Source: three-view drawing plus pictorial views. Frame: mm from the lowest corner of the part. A direction names the side the tool comes from. Coordinates: 2 decimals unless noted, no trailing zeros. Order: outer loops, then holes, each group sorted by start corner. A loop starts at its lowest first (then second) coordinate and runs counter-clockwise, first axis right, second up. Notation, with made-up numbers: (-14.75, 34.25) -> (29.25, 34.25) arc R13 ccw to (29.25, 40.25) -> close; hole circle Ø1 at (78.5, 30). An arc over 180 degrees is marked (long way). One line per question, with ' | ' between items.
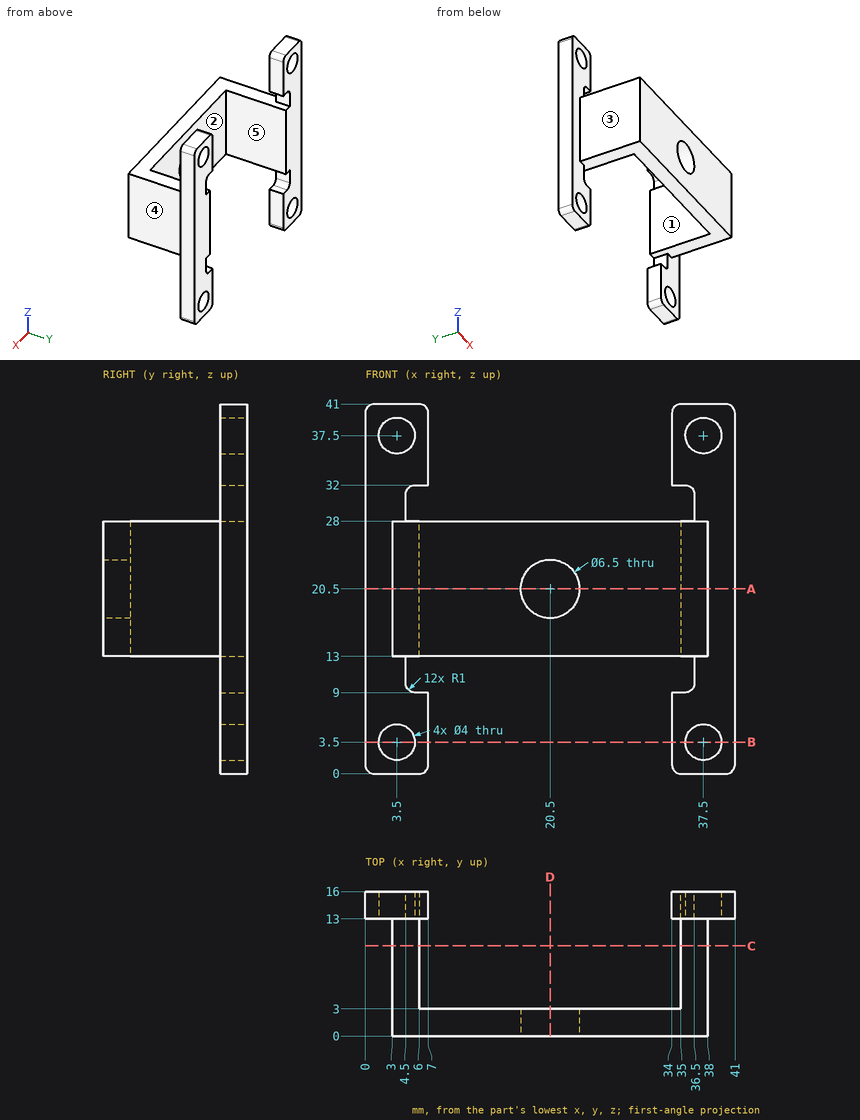
1. Cut plane C-C, the plane y = 10. Return loops of the section in (x, z).
Recorded:
outline: (3, 13) -> (6, 13) -> (6, 28) -> (3, 28) -> close; (35, 13) -> (38, 13) -> (38, 28) -> (35, 28) -> close
2. Access query for the marked faces 1, 2 and 3. Directions: +Z, -Z, +X, -X, +Y, -Y. A direction counts if a zero-diameter tool reaches every point of the face in a straight line with its end or side. Return the directions, or none.
Recorded:
face 1: +Y | face 2: +Z, -Z, +Y | face 3: +Z, -Z, -X, -Y
3. Ray query, line 1 (X direction, y = 14.8, z = 37.5); line 2 (X direction, y = 14.25, z = 20); line 3 (X direction, y = 11.75, z = 14.5). Return the intervals inside material, ascending. Write a range as [from, to].
Recorded:
line 1: x = [0, 1.5], [5.5, 7], [34, 35.5], [39.5, 41] | line 2: x = [0, 6], [35, 41] | line 3: x = [3, 6], [35, 38]
4. Cut plane D-D, the plane x = 20.5. Return loops of the section in (y, z).
Recorded:
outline: (0, 13) -> (3, 13) -> (3, 17.25) -> (0, 17.25) -> close; (0, 23.75) -> (3, 23.75) -> (3, 28) -> (0, 28) -> close
5. Cut plane A-A, the plane z = 20.5. Return loops of the section in (x, y), and give its area (4 significant figures).
Recorded:
outline: (0, 13) -> (3, 13) -> (3, 0) -> (17.25, 0) -> (17.25, 3) -> (6, 3) -> (6, 16) -> (0, 16) -> close; (23.75, 0) -> (38, 0) -> (38, 13) -> (41, 13) -> (41, 16) -> (35, 16) -> (35, 3) -> (23.75, 3) -> close | area: 181.5 mm^2
6. Pin query (flat end, axial travel): pin 1 Ø5 at (x, z) = (3.5, 3.5) entering from +Y; pin 2 Ø2 at (y, z) = (11, 9) entering from -X; pin 3 Ø6 at (x, y) = (19, 2.5) entering from -Z; pin 4 Ø16.5 at (x, z) = (22.5, 22.5) entering from +Y. Return the tip coordinate at first contact, or that it passes through.
Recorded:
pin 1: stops at y = 16 | pin 2: passes through | pin 3: stops at z = 13 | pin 4: stops at y = 3
7. Cut plane B-B, the plane z = 3.5. Return loops of the section in (x, y), and give its area (3 significant figures).
Recorded:
outline: (0, 13) -> (1.5, 13) -> (1.5, 16) -> (0, 16) -> close; (5.5, 13) -> (7, 13) -> (7, 16) -> (5.5, 16) -> close; (34, 13) -> (35.5, 13) -> (35.5, 16) -> (34, 16) -> close; (39.5, 13) -> (41, 13) -> (41, 16) -> (39.5, 16) -> close | area: 18.0 mm^2
8. Mould query, pull axis Z, two halves, no side actions, for the marked faces 4 and 5. Classes: released by +Z, released by -Z, zero draft, split by the parting line, or undercut.
Recorded:
face 4: zero draft | face 5: undercut
